```python
from build123d import *

# Parameters (mm, degrees)
SKETCH1_W           = 6.5
SKETCH1_H           = 5
BOSS_EXTRUDE1_DEPTH = 0.75
SKETCH2_R           = 1.1
CUT_EXTRUDE1_DEPTH  = 5.168333
FILLET1_R           = 0.1


with BuildPart() as part:
    # Sketch1 → Boss-Extrude1 (new body)
    with BuildSketch(Plane(origin=(0, 0, 0), x_dir=(1, 0, 0), z_dir=(0, 1, 0))):
        Rectangle(SKETCH1_W, SKETCH1_H)
    extrude(amount=BOSS_EXTRUDE1_DEPTH)

    # Sketch2 → Cut-Extrude1 (cut, through all)
    with BuildSketch(Plane(origin=(0, 0, 0), x_dir=(1, 0, 0), z_dir=(0, 1, 0))):
        with Locations(Location((0, 0.484711092, 0), (0, 0, 270))):
            Circle(SKETCH2_R)
    extrude(amount=CUT_EXTRUDE1_DEPTH, mode=Mode.SUBTRACT)

    # Fillet1
    fillet1_edges = [part.edges().sort_by_distance(p)[0] for p in [
        (-3.25, 0.75, 0),
        (0, 0.75, 2.5),
        (3.25, 0.75, 0),
        (0, 0, 2.5),
        (-3.25, 0, 0),
        (0, 0, -2.5),
        (3.25, 0, 0),
        (3.25, 0.375, 2.5),
        (-3.25, 0.375, 2.5),
        (-3.25, 0.375, -2.5),
        (3.25, 0.375, -2.5),
        (0, 0.75, -2.5),
    ]]
    fillet(fillet1_edges, radius=FILLET1_R)


solid = part.part
```
Verification items for the finished model (mm, model axes). Coordinates: 2 decimals unless noted, no trailing zeros. Loops run counter-clockwise (first coordinate to the right, second up) from the corner with the lowest first, then second, coordinate; pieces in that order, holes last. Notation, with made-up numbers: (-28, 46.25) - (-3, 46.25) arc R26 ccw to (-3, 65.25) - close; hole circle Ø10 at (36.5, 65). An arc over 180 degrees is marked (long way). Answer as a JSON object with one key per item and string values.
(1) Cross-section at A-A, the plane x = 0. Record the boundary of the cut face in (y, z), then the cut area to 3 significant figures.
Response:
{"outline": "(0, -2.4) arc R0.1 ccw to (0.1, -2.5) - (0.65, -2.5) arc R0.1 ccw to (0.75, -2.4) - (0.75, -1.58) - (0, -1.58) - close; (0, 0.62) - (0.75, 0.62) - (0.75, 2.4) arc R0.1 ccw to (0.65, 2.5) - (0.1, 2.5) arc R0.1 ccw to (0, 2.4) - close", "area": "2.09 mm²"}
(2) Cross-section at B-B, the plane z = -0.3. Record the boundary of the cut face in (x, y).
Response:
{"outline": "(-3.25, 0.1) arc R0.1 ccw to (-3.15, 0) - (-1.08, 0) - (-1.08, 0.75) - (-3.15, 0.75) arc R0.1 ccw to (-3.25, 0.65) - close; (1.08, 0) - (3.15, 0) arc R0.1 ccw to (3.25, 0.1) - (3.25, 0.65) arc R0.1 ccw to (3.15, 0.75) - (1.08, 0.75) - close"}
(3) Scan lines: line 1 along Z through (x, y) = (0, 0.5); line 2 along Z through (x, y) = (0.75, 0.15); line 3 along X through (y, z) = (0.6, -0.7). Record each from-to range of solid material in increasing order.
Response:
{"line 1": "z = -2.5 to -1.58, 0.62 to 2.5", "line 2": "z = -2.5 to -1.29, 0.32 to 2.5", "line 3": "x = -3.25 to -1.08, 1.08 to 3.25"}
(4) Mould release check, pull along Z, two halves, no side actions. Record for faces 1 (the flat face through (0, 0.75, 1)), 2 (the cylindrical face through (0.33, 0.37, 0.564)): pulls with the +Z half, pulls with the -Z half, needs draft (parallel to the pull), parting line crosses it, or undercut.
Response:
{"face 1": "needs draft", "face 2": "undercut"}
(5) Go/stop test with a flat-tipped pin: pin 1 Ø1.5 at (x, z) = (0, -1) entering from -Y. Record where the tip stops, or that it passes through.
Response:
{"pin 1": "stops at y = 0"}
(6) Cross-section at C-C, the plane y = 0.35. Record the boundary of the cut face in (x, z).
Response:
{"outline": "(-3.25, -2.4) arc R0.1 ccw to (-3.15, -2.5) - (3.15, -2.5) arc R0.1 ccw to (3.25, -2.4) - (3.25, 2.4) arc R0.1 ccw to (3.15, 2.5) - (-3.15, 2.5) arc R0.1 ccw to (-3.25, 2.4) - close; hole circle Ø2.2 at (0, -0.48)"}
